Check sheet for the drawn part. Datum: minimum x, y, z corner. Units: mm. A direction names the side the tool comes from. Give positions to 0.01 mm unless a question says otherwise; leave off trailing zeros. Loops run counter-clockwise (first coordinate to the right, second up) from the corner with the lowest first, then second, coordinate; pieces in that order, holes last. Notation, with made-up numbers: (-32.5, 27.5) - (-6.5, 27.5) arc R15 cw to (-6.5, 44.5) - close; hole circle Ø9 at (31, 50). An arc over 180 degrees is marked (long way). Use a Markdown table: item, result. Add a question column.
1. Cross-section at D-D on y = 187. Enter the section's corners in (x, z).
2. Cross-section at C-C on x = 12. Enter the section's corners in (y, z) (1 decimal).
3. Set-up check for the marked faces 1 and 2: record each of +Z, -Z, +X, -X, +Y, -Y from which the full face is reachable in a straight line by a thin tool's end or side.
4. Cross-section at A-A on z = 25. Enter the section's corners in (x, y) (1 decimal).
5. Draft check along X on the marked faces 3, 4 and 5. Enter one of: pulls with the +X half, pulls with the -X half, needs draft (parallel to the pull), parting line crosses it, or undercut.
6. Cross-section at B-B on y = 48. Enter the section's corners in (x, z).
7. Material ranges on L1, parallel to Z at x = 29, y = 147; L2, parallel to X at y = 105.5, z = 44.5; L3, parallel to X at y = 175.5, z = 27, recorded low to high.
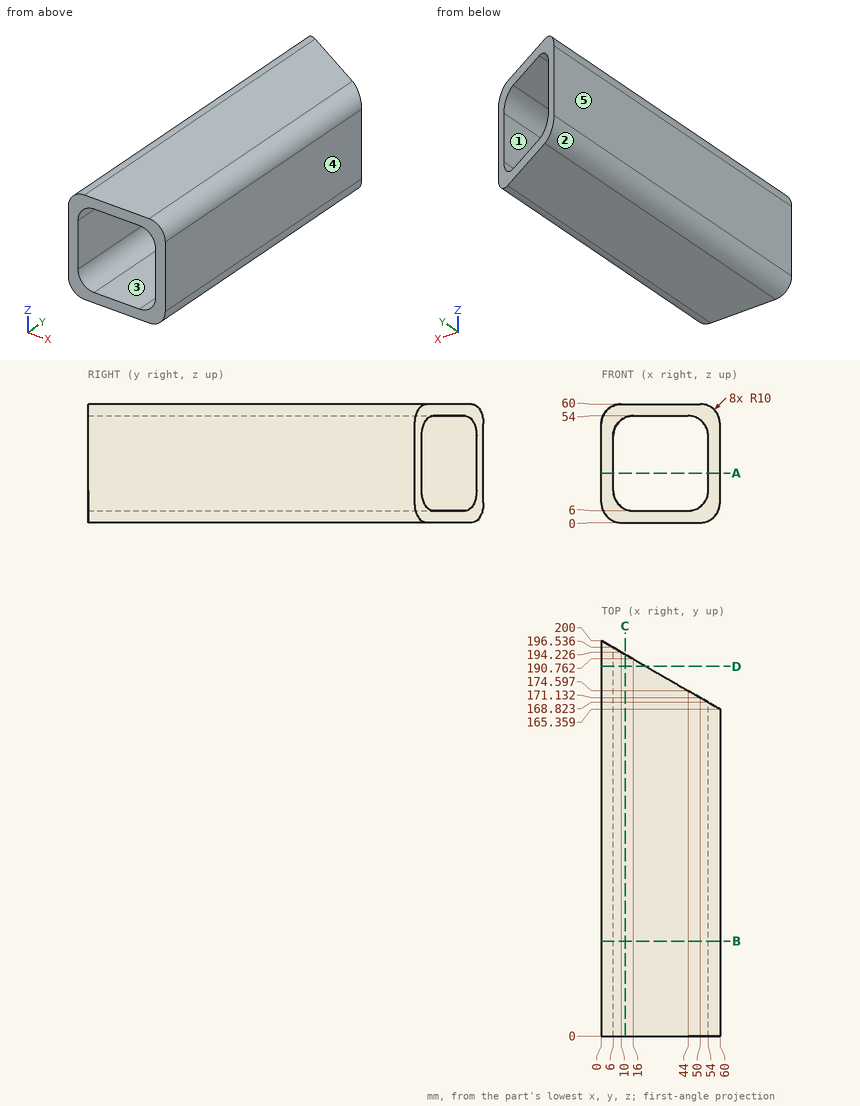
Values found:
| question | item | result |
|---|---|---|
| 1 | outline | (0, 10) arc R10 ccw to (10, 0) - (22.52, 0) - (22.52, 6) - (16, 6) arc R10 cw to (6, 16) - (6, 44) arc R10 cw to (16, 54) - (22.52, 54) - (22.52, 60) - (10, 60) arc R10 ccw to (0, 50) - close |
| 2 | outline | (0, 0) - (193.1, 0) - (193.1, 6.8) - (0, 6.8) - close; (0, 53.2) - (193.1, 53.2) - (193.1, 60) - (0, 60) - close |
| 3 | face 1 | +Y, -Y |
| 3 | face 2 | -Z, -X, +Y, -Y |
| 4 | outline | (0, 0) - (6, 0) - (6, 196.5) - (0, 200) - close; (54, 0) - (60, 0) - (60, 165.4) - (54, 168.8) - close |
| 5 | face 3 | undercut |
| 5 | face 4 | pulls with the +X half |
| 5 | face 5 | pulls with the -X half |
| 6 | outline | (0, 10) arc R10 ccw to (10, 0) - (50, 0) arc R10 ccw to (60, 10) - (60, 50) arc R10 ccw to (50, 60) - (10, 60) arc R10 ccw to (0, 50) - close; hole (6, 16) arc R10 ccw to (16, 6) - (44, 6) arc R10 ccw to (54, 16) - (54, 44) arc R10 ccw to (44, 54) - (16, 54) arc R10 ccw to (6, 44) - close |
| 7 | L1 | z = 0 to 6, 54 to 60 |
| 7 | L2 | x = 0 to 6.01, 53.99 to 60 |
| 7 | L3 | x = 0 to 6 |
